Design review of the part built by this model. Coordinates are the model's own, in mm. A direction names the side the tool comes from. Coordinates: 2 decimals unless noted, no trailing zeros. Order: outer loops, then holes, each group sorted by start corner. A loop starts at its lowest first (then second) coordinate and runs counter-clockwise, first axis right, second up. Notation, with made-up numbers: M -25,-21.5 L -8,-21.5 A18 ccw -8,6.5 Z; hole C 8.5,85.5 d1. An arc over 180 degrees is marked long. Use CSV: the item, a comma, the result in double quotes.
```python
from build123d import *

# Parameters (mm, degrees)
F0_W      = 52
F0_H      = 33
F1_DEPTH  = 8
F2_R      = 7.85
F3_DEPTH  = 7.3
F4_R      = 3.35
F5_DEPTH  = 10
F6_R      = 2
F7_W      = 2
F7_H      = 22.600369
F8_DEPTH  = 18
F9_W      = 7
F9_H      = 27
F10_DEPTH = 8.001


with BuildPart() as f1:
    # F0 (on Top) → F1 (new body)
    with BuildSketch(Plane.XY):
        with Locations((0, 0.089891)):
            Rectangle(F0_W, F0_H)
    extrude(amount=F1_DEPTH)

    # F2 (on face) → F3 (cut)
    with BuildSketch(Plane(origin=(0, 0, 0), x_dir=(1, 0, 0), z_dir=(0, 0, -1))):
        Circle(F2_R)
    extrude(amount=-F3_DEPTH, mode=Mode.SUBTRACT)

    # F4 (on face) → F5 (cut)
    with BuildSketch(Plane.XY.offset(8)):
        Circle(F4_R)
    extrude(amount=-F5_DEPTH, mode=Mode.SUBTRACT)

    # F6
    f6_edges = [f1.edges().sort_by_distance(p)[0] for p in [
        (26, -16.410109, 4),
        (26, 16.589891, 4),
        (-26, 16.589891, 4),
        (-26, -16.410109, 4),
    ]]
    fillet(f6_edges, radius=F6_R)

    # F7 (on Top) → F8 (cut)
    with BuildSketch(Plane.XY):
        with Locations((0, 11.300185)):
            Rectangle(F7_W, F7_H)
    extrude(amount=F8_DEPTH, mode=Mode.SUBTRACT)

    # F9 (on face) → F10 (cut, through all)
    with BuildSketch(Plane.XY.offset(8)):
        with Locations((-17.6, 0)):
            Rectangle(F9_W, F9_H)
        with Locations((17.6, 0)):
            Rectangle(F9_W, F9_H)
    extrude(amount=-F10_DEPTH, mode=Mode.SUBTRACT)


solid = f1.part
```
(1) The part is to be moulded in two halves that separate along X. For faces 6 (the face through (21.1, 0, 4)), 7 (the face through (25.4, 16.02, 4.06)), 8 (the face through (-6, -7, 0)), say which applies: pulls with the +X half, pulls with the -X half, needs draft (parallel to the pull), parting line crosses it, or undercut.
The answers:
face 6,"undercut"
face 7,"pulls with the +X half"
face 8,"needs draft"
(2) Clearance check with flat-ended pins moving along their axes: P1, Ø18, axis at x = 0, y = 0, coming from the -Z side; P2, Ø4.5, axis at x = 2, y = 3, coming from the -Z side. State where each tip first meets the part, or that it passes through.
The answers:
P1,"stops at z = 0"
P2,"stops at z = 7.3"
(3) Add section B-B on x = 15. State the section outline as (y, z) points.
The answers:
outline,"M -16.41,0 L -13.5,0 L -13.5,8 L -16.41,8 Z; M 13.5,0 L 16.59,0 L 16.59,8 L 13.5,8 Z"
(4) Wall thickness on probe 1 along X at (y, z) = (0, 7.5); probe 2 along X at (y, z) = (0, 3); probe 3 along X at (y, z) = (-13, 1): over which ranges is each line inside the solid? List them lowest first.
The answers:
probe 1,"x = -26 to -21.1, -14.1 to -3.35, 3.35 to 14.1, 21.1 to 26"
probe 2,"x = -26 to -21.1, -14.1 to -7.85, 7.85 to 14.1, 21.1 to 26"
probe 3,"x = -26 to -21.1, -14.1 to 14.1, 21.1 to 26"
(5) Add section A-A on y = 0. State the section outline as (x, z) points.
The answers:
outline,"M -26,0 L -21.1,0 L -21.1,8 L -26,8 Z; M -14.1,0 L -7.85,0 L -7.85,7.3 L -3.35,7.3 L -3.35,8 L -14.1,8 Z; M 3.35,7.3 L 7.85,7.3 L 7.85,0 L 14.1,0 L 14.1,8 L 3.35,8 Z; M 21.1,0 L 26,0 L 26,8 L 21.1,8 Z"
(6) Add section C-C on y = -8.5. State the section outline as (x, z) points.
The answers:
outline,"M -26,0 L -21.1,0 L -21.1,8 L -26,8 Z; M -14.1,0 L 14.1,0 L 14.1,8 L -14.1,8 Z; M 21.1,0 L 26,0 L 26,8 L 21.1,8 Z"
(7) For faces 1 (the face through (-1, 11, 4)), 2 (the face through (-21.1, 0, 4)), 3 (the face through (-25.43, -15.81, 4.06)), 4 (the face through (-26, 0, 4)), 5 (the face through (0.331, -7.843, 3.599)), list the 3-axis set-ups (+Z, -Z, +X, -X, +Y, -Y) from which the entire face can be reached by the end or side of a thin tool; tool diameter is ignored.
The answers:
face 1,"+Z, -Z, +Y"
face 2,"+Z, -Z"
face 3,"+Z, -Z, -X, -Y"
face 4,"+Z, -Z, -X, +Y, -Y"
face 5,"-Z"
(8) Add section D-D on z = 5.5. State the section outline as (x, y) points.
The answers:
outline,"M -26,-14.41 A2 ccw -24,-16.41 L 24,-16.41 A2 ccw 26,-14.41 L 26,14.59 A2 ccw 24,16.59 L 1,16.59 L 1,7.79 A7.85 cw long -1,7.79 L -1,16.59 L -24,16.59 A2 ccw -26,14.59 Z; hole M -21.1,-13.5 L -14.1,-13.5 L -14.1,13.5 L -21.1,13.5 Z; hole M 14.1,-13.5 L 21.1,-13.5 L 21.1,13.5 L 14.1,13.5 Z"
